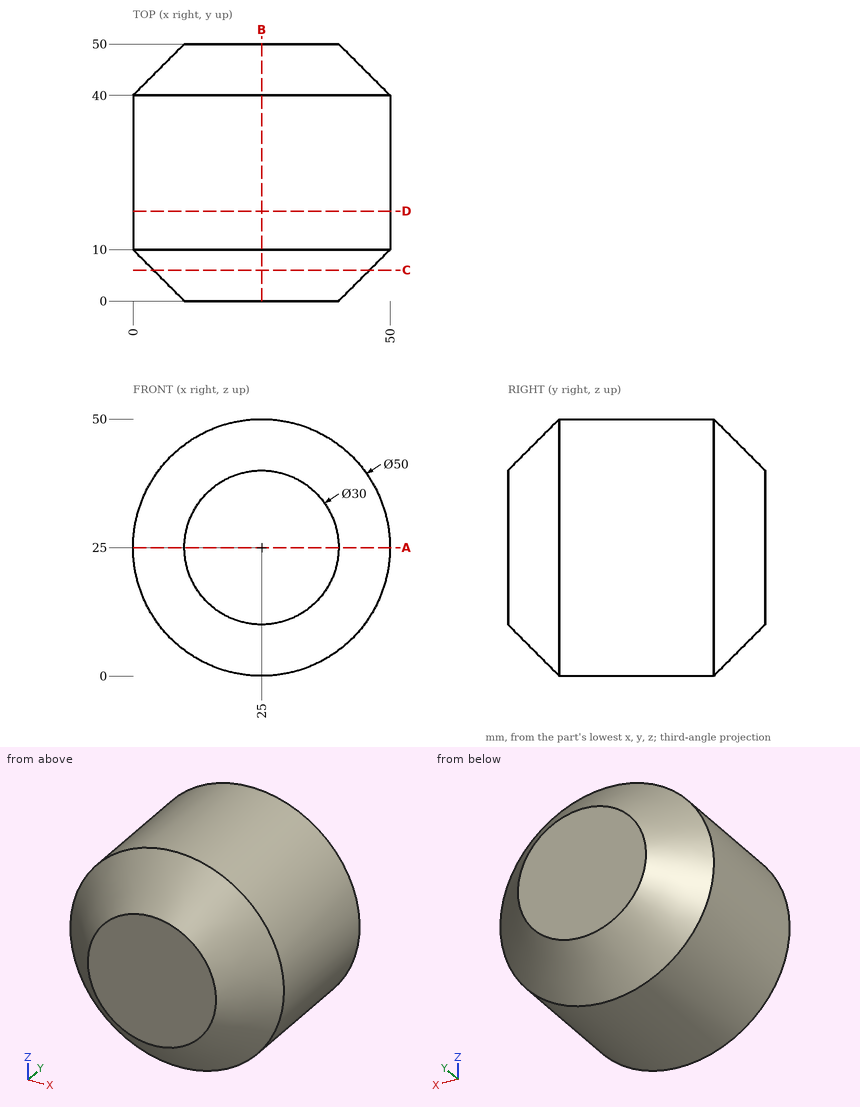
Verification items for this drawing (mm, ordinates from the low corner). Round coordinates to 2 decimals unless told otherwise and drop trailing zeros. Loops run counter-clockwise (first coordinate to the right, second up) from the corner with the lowest first, then second, coordinate; pieces in that order, holes last. Notation, with made-up numbers: (-36, -30) -> (-3, -30) arc R21 cw to (-3, -17) -> close; hole circle Ø5 at (70.5, -29). An arc over 180 degrees is marked (long way). Write item = value, one per line. Start each with the question number.
1) Thickness scan on probe 1 along X at (y, z) = (41, 16.5); probe 2 along Z at (x, y) = (26, 37); probe 3 along Y at (x, z) = (11.5, 12). Record the ranges inside material, lowest first.
2) Sectioned sample at A-A, the plane z = 25. Record the cut outline in (x, y), plus the area to 3 significant figures.
3) Sectioned sample at D-D, the plane y = 17.5. Record the cut outline in (x, z).
4) Sectioned sample at C-C, the plane y = 6. Record the cut outline in (x, z), plus the area to 3 significant figures.
5) Gauge pin test, flat ends, axial feed: pin 1 Ø8 at (y, z) = (25.5, 36.5) entering from +X; pin 2 Ø1.5 at (y, z) = (16.5, 25.5) entering from -X; pin 3 Ø4 at (y, z) = (30.5, 12.5) entering from -X; pin 4 Ø8 at (x, y) = (23.5, 27) entering from +Z. Record the tip position at first contact, or that the pin passes through.
Results are:
q1.probe_1 = 2.56 to 47.44
q1.probe_2 = 0.02 to 49.98
q1.probe_3 = 3.74 to 46.26
q2.outline = (0, 10) -> (10, 0) -> (40, 0) -> (50, 10) -> (50, 40) -> (40, 50) -> (10, 50) -> (0, 40) -> close
q2.area = 2,300 mm^2
q3.outline = circle Ø50 at (25, 25)
q4.outline = circle Ø42 at (25, 25)
q4.area = 1,390 mm^2
q5.pin_1 = 48.85
q5.pin_2 = 0
q5.pin_3 = 2.31
q5.pin_4 = 50
